```python
from build123d import *

# Parameters (mm, degrees)
BOSS_EXTRUDE1_DEPTH = 5
BOSS_EXTRUDE2_DEPTH = 1
BOSS_EXTRUDE3_DEPTH = 1


with BuildPart() as part:
    # Sketch1 → Boss-Extrude1 (new body)
    with BuildSketch(Plane(origin=(0, 0, 0), x_dir=(1, 0, 0), z_dir=(0, 1, 0))):
        Polygon((-82.55, -63.5), (-82.55, -86.36), (-76.2, -86.36), (-76.2, -63.5), (76.2, -63.5), (76.2, -86.36), (82.55, -86.36), (82.55, 86.36), (76.2, 86.36), (76.2, 63.5), (-76.2, 63.5), (-76.2, 86.36), (-82.55, 86.36), (-82.55, 63.5), (-119.360030459, 63.5), (-119.360030459, -63.5), align=None)
    extrude(amount=BOSS_EXTRUDE1_DEPTH)

    # Sketch4 → Cut-Revolve3 (revolve, cut)
    with BuildSketch(Plane(origin=(-76.2, 0, 0), x_dir=(0, 0, -1), z_dir=(1, 0, 0))):
        with BuildLine():
            Line((-82.55, 4.5), (-82.55, 0.5))
            ThreePointArc((-82.55, 0.5), (-80.55, 2.5), (-82.55, 4.5))
        make_face()
    revolve(axis=Axis((-76.2, 4.5, 82.55), (0, -1, 0)), mode=Mode.SUBTRACT)

    # Sketch5 → Cut-Revolve4 (revolve, cut)
    with BuildSketch(Plane.ZY.offset(-76.2)):
        with BuildLine():
            Line((82.55, 0.5), (82.55, 4.5))
            ThreePointArc((82.55, 4.5), (84.55, 2.5), (82.55, 0.5))
        make_face()
    revolve(axis=Axis((76.2, 0.5, 82.55), (0, 1, 0)), mode=Mode.SUBTRACT)

    # Sketch7 → Loft1 section 0
    with BuildSketch(Plane(origin=(0, 5, 0), x_dir=(1, 0, 0), z_dir=(0, 1, 0))):
        with BuildLine():
            Line((-26.67, -63.5), (26.67, -63.5))
            Line((26.67, -63.5), (26.67, 63.5))
            Line((26.67, 63.5), (-26.67, 63.5))
            Line((-26.67, 63.5), (-26.67, -63.5))
        make_face()
    # Sketch6 → Loft1 section 1
    with BuildSketch(Plane(origin=(0, 19.05, 0), x_dir=(1, 0, 0), z_dir=(0, 1, 0))):
        with BuildLine():
            Line((26.67, 1.27), (-26.67, 1.27))
            Line((-26.67, 1.27), (-26.67, -1.27))
            Line((-26.67, -1.27), (26.67, -1.27))
            Line((26.67, -1.27), (26.67, 1.27))
        make_face()
    loft()

    # Sketch8 → Cut-Revolve5 (revolve, cut)
    with BuildSketch(Plane(origin=(-76.2, 0, 0), x_dir=(0, 0, -1), z_dir=(1, 0, 0))):
        with BuildLine():
            Line((82.55, 4.5), (82.55, 0.5))
            ThreePointArc((82.55, 0.5), (84.55, 2.5), (82.55, 4.5))
        make_face()
    revolve(axis=Axis((-76.2, 4.5, -82.55), (0, -1, 0)), mode=Mode.SUBTRACT)

    # Sketch9 → Cut-Revolve6 (revolve, cut)
    with BuildSketch(Plane.ZY.offset(-76.2)):
        with BuildLine():
            Line((-82.55, 4.405), (-82.55, 0.595))
            ThreePointArc((-82.55, 0.595), (-80.645, 2.5), (-82.55, 4.405))
        make_face()
    revolve(axis=Axis((76.2, 4.405, -82.55), (0, -1, 0)), mode=Mode.SUBTRACT)

    # Sketch10 → Boss-Extrude2 (add)
    with BuildSketch(Plane(origin=(26.67, 0, 0), x_dir=(0, 0, -1), z_dir=(1, 0, 0))):
        Polygon((-63.5, 5), (63.5, 5), (72.033936378, 21.05), (-72.033936378, 21.05), align=None)
    extrude(amount=BOSS_EXTRUDE2_DEPTH)

    # Sketch11 → Boss-Extrude3 (add)
    with BuildSketch(Plane.ZY.offset(26.67)):
        Polygon((-63.5, 5), (63.5, 5), (72.033936378, 21.05), (-72.033936378, 21.05), align=None)
    extrude(amount=BOSS_EXTRUDE3_DEPTH)


solid = part.part
```
Geometry: final body of the model. Coordinates: model frame, mm. A direction names the side the tool comes from. Round coordinates to 2 decimals unless told otherwise and drop trailing zeros. Write each loop counter-clockwise with the first axis right and the second up, starting at its lowest first coordinate (ties: lowest second). Pieces come first, ordered by that corner, then holes. Notation, with made-up numbers: M 66,51.5 L 89,51.5 A30 ccw 89,77.5 Z; hole C 19,26.5 d3. An arc over 180 degrees is marked long. Answer in a Markdown table with one row per item. Add a question column.
(1) Cut plane C-C, the plane z = 22. Return the cut outline in (x, y).
(2) Cut plane B-B, the plane y = 12.5. Return the cut outline in (x, z).
(3) Cut plane A-A, the plane x = -7. Return the cut outline in (y, z), then the cut area to 3 significant figures.
(4) Reachability of faces 5 (the face through (-74, 5, -1)), 6 (the face through (-101, 2, 63.5)), 7 (the face through (-76.2, 2, -75)), 8 (the face through (-101, 2, -63.5)) from +Z, -Z, +X, -X, +Y, -Y: full face, straight path, thin tool, end or side. Return the list, or none.
(5) Contact query for flat-ended pins moving along their axis: pin 1 (8 mm diameter, centred on y = 16.5, z = -65.5, fed in from +X); pin 2 (12 mm diameter, centred on y = 10, z = 9, fed in from +X); pin 3 (4 mm diameter, centred on x = -8.5, y = 1.5, fed in from +Z); pin 4 (10 mm diameter, centred on x = -64.5, y = 11, fed in from -Z). Output: stop coordinate, or through.
(6) Cut plane D-D, the plane x = 48.5. Return the cut outline in (y, z), then the cut area to 3 significant figures.
(7) Draft query along X for faces 1 (the face through (76.2, 2, -75)), 2 (the face through (-0.373, 12.123, 31.949)), 3 (the face through (-119.36, 2, -1)), 4 (the face through (55, 5, -1)). Return one class per face: pulls with the +X half, pulls with the -X half, needs draft (parallel to the pull), parting line crosses it, or undercut.
(8) Ray query, L1, parallel to X at y = 16.75, z = -58.5; L2, parallel to Y at x = -85.5, z = -16.5; L3, parallel to Z at x = 5.5, y = 1.75. Return the intervals inside material, ascending.
Established:
| question | item | result |
|---|---|---|
| 1 | outline | M -119.36,0 L 82.55,0 L 82.55,5 L 27.67,5 L 27.67,21.05 L 26.67,21.05 L 26.67,14.37 L -26.67,14.37 L -26.67,21.05 L -27.67,21.05 L -27.67,5 L -119.36,5 Z |
| 2 | outline | M -27.67,-67.49 L -26.67,-67.49 L -26.67,-30.28 L 26.67,-30.28 L 26.67,-67.49 L 27.67,-67.49 L 27.67,67.49 L 26.67,67.49 L 26.67,30.28 L -26.67,30.28 L -26.67,67.49 L -27.67,67.49 Z |
| 3 | outline | M 0,-63.5 L 5,-63.5 L 19.05,-1.27 L 19.05,1.27 L 5,63.5 L 0,63.5 Z |
| 3 | area | 1,550 mm² |
| 4 | face 5 | +Z, -Z, -X, +Y |
| 4 | face 6 | +Z, -X, +Y, -Y |
| 4 | face 7 | -Z, +Y, -Y |
| 4 | face 8 | -Z, -X, +Y, -Y |
| 5 | pin 1 | x = 27.67 |
| 5 | pin 2 | x = 82.55 |
| 5 | pin 3 | z = 63.5 |
| 5 | pin 4 | through |
| 6 | outline | M 0,-63.5 L 5,-63.5 L 5,63.5 L 0,63.5 Z |
| 6 | area | 635 mm² |
| 7 | face 1 | undercut |
| 7 | face 2 | undercut |
| 7 | face 3 | pulls with the -X half |
| 7 | face 4 | needs draft |
| 8 | L1 | -27.67 to -26.67, 26.67 to 27.67 |
| 8 | L2 | 0 to 5 |
| 8 | L3 | -63.5 to 63.5 |
